Build history of the part. All positions in model axes, mm. Face numbers are marked on the shaded views. Round coordinates to 2 decimals unless told otherwise and drop trailing zeros. Loops run counter-clockwise (first coordinate to the right, second up) from the corner with the lowest first, then second, coordinate; pieces in that order, holes last. Notation, with made-up numbers: (69, 14) - (81, 14) arc R22 ccw to (81, 35) - close; hole circle Ø6 at (64.5, 18.25). An arc over 180 degrees is marked (long way). Use one line per item in the form item = value. Start each with the question number.
Q1. Saw through at C-C (y = 0). Count the separate pieces of the cut face and the enclosed holes in it, then the cut area to 3 significant figures.
Q2. Saw through at A-A (z = -0.75). Give the cut face in (x, y).
Q3. Saw through at D-D (z = -5.25). Give the cut face in (x, y), then the cut area to 3 significant figures.
Q4. Mould opens along Z. For the marked faces 1, 2 and 3 say: released by +Z, released by -Z, zero draft, split by the parting line, or undercut.
Q5. Drill centre lines: line 1 (X direction, y = -0.25, z = 0); line 2 (Y direction, x = -3, z = -0.25); line 3 (X direction, y = -2.25, z = -8.5). Where is each one in solid material? Low to high.
Q6. Saw through at B-B (x = 10). Give the cut face in (y, z), then the cut area to 3 significant figures.
Q7. Pin check, flat tips, straight feed: pin 1 (1.5 mm diameter, centred on x = -18.5, z = -8.5, fed in from -Y); pin 2 (4 mm diameter, centred on x = -12, z = 0, fed in from -Y); pin 3 (1 mm diameter, centred on x = 4.5, z = 8, fed in from -Y); pin 4 (4 mm diameter, centred on x = 17.5, z = 3.5, fed in from -Y). Stop position of each tip, or through.
Autodesk Inventor part; units mm, degrees
ref_plane "YZ Plane" through (0, 0, 0) normal (1, 0, 0) x (0, 1, 0)
ref_plane "XZ Plane" through (0, 0, 0) normal (0, 1, 0) x (-1, 0, 0)
ref_plane "XY Plane" through (0, 0, 0) normal (0, 0, 1) x (1, 0, 0)
sketch "Sketch1" plane through (0, 0, 0) normal (0, 1, 0) x (-1, 0, 0)
  line L0 (-20, 10) -> (20, 10)
  line L1 (20, 10) -> (20, -10)
  line L2 (20, -10) -> (-20, -10)
  line L3 (-20, -10) -> (-20, 10)
  line L4 (-20, 10) -> (20, -10) construction
  line L5 (20, 10) -> (-20, -10) construction
  point P0 (0, 0)
  dimension "d2" = 40
  dimension "d3" = 20
extrude "Extrusion1" add sketch "Sketch1" along normal mid plane 2
sketch "Sketch5" plane through (0, -1, 0) normal (0, -1, 0) x (1, 0, 0)
  line L0 (20, 10) -> (15, 10)
  line L1 (15, 10) -> (15, -10)
  line L2 (15, -10) -> (20, -10)
  line L3 (20, -10) -> (20, 10)
  line L4 (20, 10) -> (-20, 10)
  line L5 (20, -10) -> (20, 10)
  line L6 (-20, -10) -> (20, -10)
  dimension "d25" = 5
extrude "Extrusion4" add sketch "Sketch5" along normal blind 5
sketch "Sketch4" plane through (0, -6, 0) normal (0, -1, 0) x (1, 0, 0)
  circle A0 centre (17.5, 7.5) radius 0.95
  circle A1 centre (17.5, -7.5) radius 0.95
  line L0 (20, -10) -> (20, 10)
  line L1 (20, 10) -> (15, 10)
  line L2 (15, -10) -> (20, -10)
  dimension "d26" = 1.9
  dimension "d27" = 1.9
  dimension "d28" = 2.5
  dimension "d29" = 2.5
  dimension "d30" = 2.5
extrude "Extrusion3" add sketch "Sketch4" along normal blind 2
sketch "Sketch6" plane through (0, -1, 0) normal (0, -1, 0) x (1, 0, 0)
  circle A0 centre (-18.5, 8) radius 0.95
  circle A1 centre (-18.5, -8) radius 0.95
  line L0 (-20, 10) -> (-20, -10)
  line L1 (15, 10) -> (-20, 10)
  line L2 (-20, -10) -> (15, -10)
  point P0 (0, 0)
  dimension "d31" = 1.9
  dimension "d32" = 1.9
  dimension "d33" = 1.5
  dimension "d34" = 2
  dimension "d35" = 2
extrude "Extrusion5" add sketch "Sketch6" along normal blind 2
fillet "Fillet1" radius 2 4 edges at (20, -2.5, 10) (20, -2.5, -10) (-20, 0, 10) (-20, 0, -10)
sketch "Sketch7" plane through (0, 1, 0) normal (0, 1, 0) x (1, 0, 0)
  circle A0 centre (4.677, 0) radius 3.9688
  circle A1 centre (4.677, 0) radius 6.75
  point P0 (0, 0)
  dimension "d38" = 13.5
extrude "Extrusion6" cut sketch "Sketch7" against normal through all contours A0 | A1
sketch "Sketch8" plane through (0, 1, 0) normal (0, 1, 0) x (1, 0, 0)
  circle A0 centre (-12, 0) radius 2.1525
  point P0 (0, 0)
hole "Hole1" at (-12, 1, 0) direction (0, -1, 0) diameter 4.305 end through all
equation "\"d27\" = d26"
equation "\"d29\" = d28"
equation "\"d30\" = d29"
equation "\"d32\" = d31"
equation "\"d35\" = d34"
properties part number "GearCover"
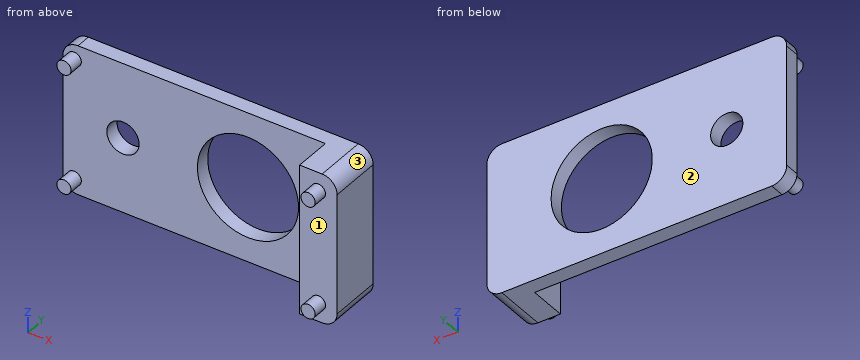
Report:
q1.separate_pieces = 1
q1.enclosed_holes = 2
q1.area = 639 mm²
q2.outline = (-20, -1) - (-14.02, -1) - (-14.02, 1) - (-20, 1) - close; (-9.98, -1) - (-2.03, -1) - (-2.03, 1) - (-9.98, 1) - close; (11.39, -1) - (15, -1) - (15, -6) - (20, -6) - (20, 1) - (11.39, 1) - close
q3.outline = (-20, -1) - (0.43, -1) - (0.43, 1) - (-20, 1) - close; (8.92, -1) - (15, -1) - (15, -6) - (20, -6) - (20, 1) - (8.92, 1) - close
q3.area = 88.0 mm²
q4.face_1 = undercut
q4.face_2 = zero draft
q4.face_3 = released by +Z
q5.line_1 = -20 to -14.15, -9.85 to -2.07, 11.43 to 20
q5.line_2 = -1 to 1
q5.line_3 = -19.31 to -17.69, 15 to 19.94
q6.outline = (-1, -10) - (1, -10) - (1, -4.15) - (-1, -4.15) - close; (-1, 4.15) - (1, 4.15) - (1, 10) - (-1, 10) - close
q6.area = 23.4 mm²
q7.pin_1 = -3
q7.pin_2 = through
q7.pin_3 = -1
q7.pin_4 = -6
